```python
from build123d import *

# Parameters (mm, degrees)
BOSS_EXTRUDE10_DEPTH = 1.27


with BuildPart() as part:
    # Sketch1 → Boss-Extrude10 (new, symmetric)
    with BuildSketch(Plane(origin=(0, 0, 0), x_dir=(1, 0, 0), z_dir=(0, 1, 0))):
        with BuildLine():
            Line((-40.034645199, 5.723587865), (-5.476888276, 5.723587865))
            Line((-5.476888276, 5.723587865), (-5.476888276, 26.661855827))
            ThreePointArc((-5.476888276, 26.661855827), (-4.732939501, 28.457907051), (-2.936888276, 29.201855827))
            Line((-2.936888276, 29.201855827), (2.631615538, 29.201855827))
            ThreePointArc((2.631615538, 29.201855827), (4.427666762, 28.457907051), (5.171615538, 26.661855827))
            Line((5.171615538, 26.661855827), (5.171615538, 5.723587865))
            Line((5.171615538, 5.723587865), (40.023244529, 5.723587865))
            ThreePointArc((40.023244529, 5.723587865), (45.741799588, 0.005032806), (40.023244529, -5.713522253))
            Line((40.023244529, -5.713522253), (-40.034645199, -5.713522253))
            ThreePointArc((-40.034645199, -5.713522253), (-45.753200258, 0.005032806), (-40.034645199, 5.723587865))
        make_face()
        with BuildLine():
            Line((-40.034645199, 2.362682699), (40.023244529, 2.362682699))
            ThreePointArc((40.023244529, 2.362682699), (42.380894421, 0.005032806), (40.023244529, -2.352617087))
            Line((40.023244529, -2.352617087), (-40.034645199, -2.352617087))
            ThreePointArc((-40.034645199, -2.352617087), (-42.392295092, 0.005032806), (-40.034645199, 2.362682699))
        make_face(mode=Mode.SUBTRACT)
        with BuildLine():
            Line((-3.238670488, 5.723587865), (2.946447825, 5.723587865))
            Line((2.946447825, 5.723587865), (2.946447825, 25.391855827))
            ThreePointArc((2.946447825, 25.391855827), (2.574473437, 26.289881439), (1.676447825, 26.661855827))
            Line((1.676447825, 26.661855827), (-1.968670488, 26.661855827))
            ThreePointArc((-1.968670488, 26.661855827), (-2.8666961, 26.289881439), (-3.238670488, 25.391855827))
            Line((-3.238670488, 25.391855827), (-3.238670488, 5.723587865))
        make_face(mode=Mode.SUBTRACT)
    extrude(amount=BOSS_EXTRUDE10_DEPTH, both=True)


solid = part.part
```
Input: part model. Units: mm. Frame: model coordinates. A direction names the side the tool comes from. Round coordinates to 2 decimals unless told otherwise and drop trailing zeros. Write each loop counter-clockwise with the first axis right and the second up, starting at its lowest first coordinate (ties: lowest second). Pieces come first, ordered by that corner, then holes. Notation, with made-up numbers: (10, 81.5) -> (18, 81.5) arc R23 ccw to (18, 104.5) -> close; hole circle Ø11 at (3.25, 28). An arc over 180 degrees is marked (long way). Answer as CSV lines item,"result".
1. Section C-C (y = 0.85). Return the cut outline in (x, z), plus the area to 3 significant figures.
Geometry says:
outline,"(-40.03, -5.72) -> (-5.48, -5.72) -> (-5.48, -26.66) arc R2.54 ccw to (-2.94, -29.2) -> (2.63, -29.2) arc R2.54 ccw to (5.17, -26.66) -> (5.17, -5.72) -> (40.02, -5.72) arc R5.72 ccw to (40.02, 5.71) -> (-40.03, 5.71) arc R5.72 ccw to start; hole (-40.03, -2.36) -> (40.02, -2.36) arc R2.36 ccw to (40.02, 2.35) -> (-40.03, 2.35) arc R2.36 ccw to start; hole (-3.24, -25.39) arc R1.27 ccw to (-1.97, -26.66) -> (1.68, -26.66) arc R1.27 ccw to (2.95, -25.39) -> (2.95, -5.72) -> (-3.24, -5.72) -> close"
area,"742 mm^2"
2. Section A-A (z = -20.5). Return the cut outline in (x, y).
Geometry says:
outline,"(-5.48, -1.27) -> (-3.24, -1.27) -> (-3.24, 1.27) -> (-5.48, 1.27) -> close; (2.95, -1.27) -> (5.17, -1.27) -> (5.17, 1.27) -> (2.95, 1.27) -> close"
3. Ray query, L1, parallel to Z at x = -1, y = 0.55; L2, parallel to Z at x = 21, y = 0.45; L3, parallel to X at y = 0, z = -24.5. Return the intervals inside material, ascending. Write a range as [from, to].
Geometry says:
L1,"z = [-29.2, -26.66], [-5.72, -2.36], [2.35, 5.71]"
L2,"z = [-5.72, -2.36], [2.35, 5.71]"
L3,"x = [-5.48, -3.24], [2.95, 5.17]"
4. Section B-B (x = 21). Return the cut outline in (y, z).
Geometry says:
outline,"(-1.27, -5.72) -> (1.27, -5.72) -> (1.27, -2.36) -> (-1.27, -2.36) -> close; (-1.27, 2.35) -> (1.27, 2.35) -> (1.27, 5.71) -> (-1.27, 5.71) -> close"
5. Reachability of faces 1 (the flat face through (-5.477, 0, -16)), 2 (the flat face through (22, 0, -5.724)), 3 (the flat face through (1, 0, 5.714)), 4 (the flat face through (0, 1.27, -3)), 5 (the flat face through (2.946, 0, -15)) from +Z, -Z, +X, -X, +Y, -Y: full face, straight path, thin tool, end or side. Return the list, or none.
Geometry says:
face 1,"-Z, -X, +Y, -Y"
face 2,"-Z, +X, +Y, -Y"
face 3,"+Z, +X, -X, +Y, -Y"
face 4,"+Z, -Z, +X, -X, +Y"
face 5,"+Y, -Y"
6. Mould query, pull axis X, two halves, no side actions, for faces 6 (the flat face through (0, 0, -5.724)), 7 (the flat face through (-23, 0, -5.724)), 8 (the flat face through (5.172, 0, -16)), 9 (the cylindrical face through (-42.39, 0.02, 0.05)). Classes: +X half, -X half, draft (parallel to the pull), parting line (faces both ways), or undercut.
Geometry says:
face 6,"undercut"
face 7,"draft"
face 8,"+X half"
face 9,"undercut"
7. Contact query for a flat-ended pin moving along its axis: P1, Ø1.3, axis at x = 8.5, y = 0, coming from the -Z side. Output: stop coordinate, or through.
Geometry says:
P1,"stops at z = -5.72"
